The model under review builds one solid part; all positions refer to its coordinate system, in mm. Face numbers are marked on the shaded views. A direction names the side the tool comes from. Give positions to 0.01 mm unless a question says otherwise; leave off trailing zeros. Loops run counter-clockwise (first coordinate to the right, second up) from the corner with the lowest first, then second, coordinate; pieces in that order, holes last. Notation, with made-up numbers: (86, 12.5) - (134, 12.5) arc R17 ccw to (134, 37.5) - close; hole circle Ø11 at (14.25, 67.25). An arc over 180 degrees is marked (long way). Answer as a JSON object with one key per item and string values.
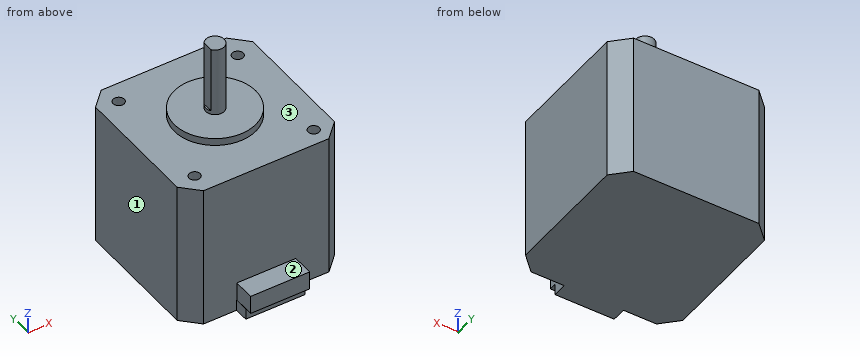
Solid Edge part; units mm, degrees
sketch "Sketch1" plane through (0, 0, 0) normal (0, 0, 1) x (1, 0, 0)
  line L0 (-16.9338, 21.25) -> (16.9338, 21.25)
  line L1 (16.9338, 21.25) -> (21.25, 16.9338)
  line L2 (21.25, 16.9338) -> (21.25, -16.9338)
  line L3 (16.9338, -21.25) -> (21.25, -16.9338)
  line L4 (16.9338, -21.25) -> (-16.9338, -21.25)
  line L5 (-21.25, -16.9338) -> (-16.9338, -21.25)
  line L6 (-21.25, -16.9338) -> (-21.25, 16.9338)
  line L7 (-21.25, 16.9338) -> (-16.9338, 21.25)
  dimension "D1" = 21.25
  dimension "D2" = 16.9338
extrude "Protrusion1" add sketch "Sketch1" along normal blind 39.2
sketch "Sketch2" plane through (0, 0, 0) normal (0, 0, 1) x (1, 0, 0)
  line L0 (0, -25.05) -> (8, -25.05)
  line L1 (8, -25.05) -> (8, -21.25)
  line L2 (8, -21.25) -> (-8, -21.25)
  line L3 (-8, -21.25) -> (-8, -25.05)
  line L4 (-8, -25.05) -> (0, -25.05)
extrude "ExtrudedProtrusion_2" add sketch "Sketch2" along normal blind 3
sketch "Sketch3" plane through (0, -23.15, 3) normal (0, 0, 1) x (1, 0, 0)
  line L0 (0, -3.8049) -> (8, -3.8049)
  line L1 (8, -3.8049) -> (8, 1.9)
  line L2 (8, 1.9) -> (-7.9332, 1.9)
  line L3 (-7.9332, 1.9) -> (-7.9332, -3.8049)
  line L4 (-7.9332, -3.8049) -> (0, -3.8049)
extrude "ExtrudedProtrusion_3" add sketch "Sketch3" along normal blind 5
sketch "Sketch4" plane through (0, 0, 39.2) normal (0, 0, 1) x (1, 0, 0)
  circle A0 centre (0, 0) radius 11
extrude "ExtrudedProtrusion_4" add sketch "Sketch4" along normal blind 2
sketch "Sketch5" plane through (0, 0, 39.2) normal (0, 0, 1) x (1, 0, 0)
  circle A0 centre (0, 0) radius 2.5
extrude "ExtrudedProtrusion_5" add sketch "Sketch5" along normal blind 21
sketch "Sketch6" plane through (0, 0, 60.2) normal (0, 0, 1) x (1, 0, 0)
  line L0 (-2.05, 2.7947) -> (-2.05, -2.6865)
  line L1 (-3.2935, -2.0855) -> (-2.05, -2.6865)
  line L2 (-4.0147, 1.8811) -> (-3.2935, -2.0855)
  line L3 (-2.05, 2.7947) -> (-4.0147, 1.8811)
extrude "ExtrudedCutout_1" cut sketch "Sketch6" against normal blind 18
hole "Hole_1" at (-15.75, 15.75, 39.2) direction (0, 0, -1) diameter 3 depth 5 tip angle 118
hole "Hole1" at (15.75, 14.75, 39.2) direction (0, 0, -1) diameter 3 depth 5 tip angle 118
hole "Hole2" at (15.75, -16.75, 39.2) direction (0, 0, -1) diameter 3 depth 5 tip angle 118
hole "Hole3" at (-15.75, -15.75, 39.2) direction (0, 0, -1) diameter 3 depth 5 tip angle 118
Q1. To check wall thickness, follow probe 1 along Y at (x, z) = (15.75, 38.2); probe 2 along X at (y, z) = (15, 35); probe 3 along Z at (x, y) = (14, 9). State the ranges of each line that lie inside material, in increasing order. Write a range as [from, to].
Results:
{"probe 1": "y = [-21.25, -18.25], [-15.25, 13.25], [16.25, 21.25]", "probe 2": "x = [-21.25, -17.05], [-14.45, 14.27], [17.23, 21.25]", "probe 3": "z = [0, 39.2]"}
Q2. Clearance check with flat-ended pins moving along their axes: pin 1 Ø3 at (x, y) = (3, -24) entering from +Z; pin 2 Ø0.9 at (y, z) = (0, 47.5) entering from -X; pin 3 Ø11 at (x, y) = (3, 0) entering from +Z; pin 4 Ø0.5 at (x, y) = (-2.5, -0.5) entering from +Z. State where each tip first meets the part, or that it passes through.
Results:
{"pin 1": "stops at z = 8", "pin 2": "stops at x = -2.05", "pin 3": "stops at z = 60.2", "pin 4": "stops at z = 42.2"}
Q3. Consider section A-A, the plane z = 27. State the section outline as (x, y) points, plus the area to 3 significant figures.
Results:
{"outline": "(-21.25, -16.93) - (-16.93, -21.25) - (16.93, -21.25) - (21.25, -16.93) - (21.25, 16.93) - (16.93, 21.25) - (-16.93, 21.25) - (-21.25, 16.93) - close", "area": "1,770 mm^2"}
Q4. Consider section D-D, the plane z = 5.5. State the section outline as (x, y) points.
Results:
{"outline": "(-21.25, -16.93) - (-16.93, -21.25) - (-7.93, -21.25) - (-7.93, -26.95) - (8, -26.95) - (8, -21.25) - (16.93, -21.25) - (21.25, -16.93) - (21.25, 16.93) - (16.93, 21.25) - (-16.93, 21.25) - (-21.25, 16.93) - close"}
Q5. Consider section C-C, the plane y = -12. State the section outline as (x, z) points, plus the area to 3 significant figures.
Results:
{"outline": "(-21.25, 0) - (21.25, 0) - (21.25, 39.2) - (-21.25, 39.2) - close", "area": "1,670 mm^2"}
Q6. Consider section B-B, the plane x = 0. State the section outline as (y, z) points, plus the area to 3 significant figures.
Results:
{"outline": "(-26.95, 3) - (-25.05, 3) - (-25.05, 0) - (21.25, 0) - (21.25, 39.2) - (11, 39.2) - (11, 41.2) - (2.5, 41.2) - (2.5, 60.2) - (-2.5, 60.2) - (-2.5, 41.2) - (-11, 41.2) - (-11, 39.2) - (-21.25, 39.2) - (-21.25, 8) - (-26.95, 8) - close", "area": "1,840 mm^2"}
Q7. For the marked faces 1, 2 and 3, list the 3-axis set-ups (+Z, -Z, +X, -X, +Y, -Y) from which the entire face can be reached by the end or side of a thin tool; tool diameter is ignored.
Results:
{"face 1": "+Z, -Z, -X, +Y, -Y", "face 2": "+Z, +X, -X, -Y", "face 3": "+Z"}
